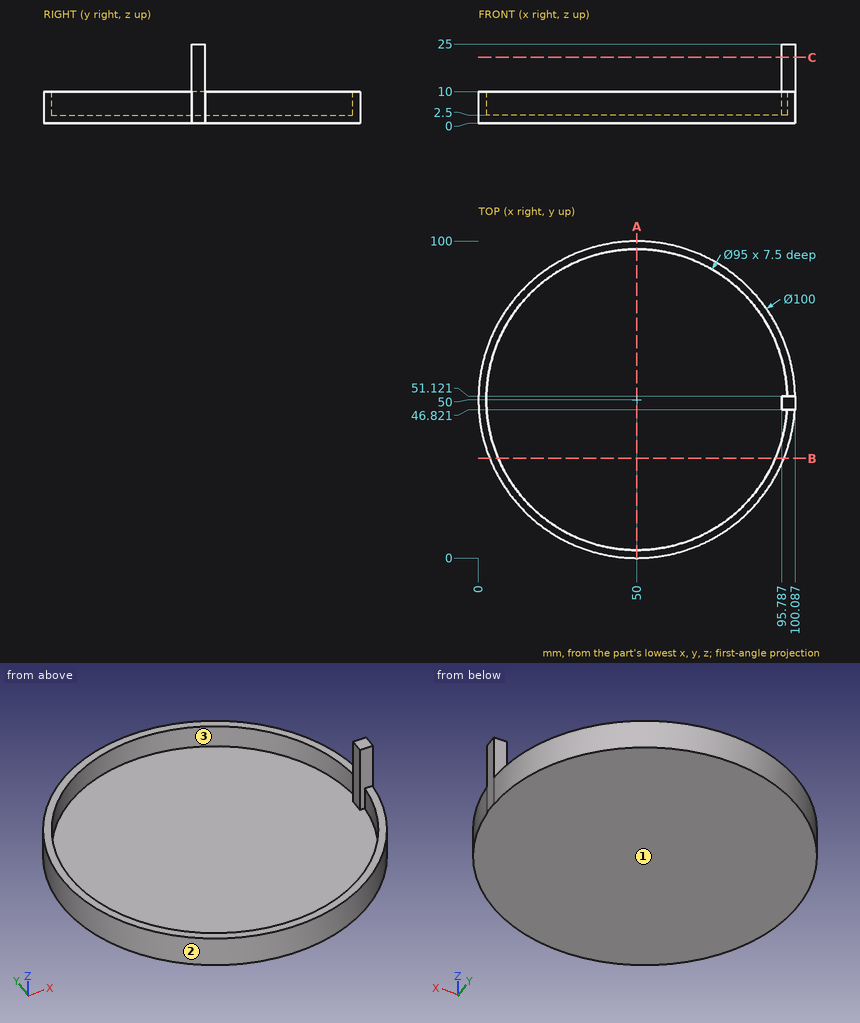
Job drawing, mm, ordinate dimensions from the low corner. One solid piece. Give positions to 0.01 mm unless a question says otherwise; leave off trailing zeros. Order: outer loops, then holes, each group sorted by start corner. A loop starts at its lowest first (then second) coordinate and runs counter-clockwise, first axis right, second up. Notation, with made-up numbers: (52, 41) -> (89, 41) arc R26 ccw to (89, 57) -> close; hole circle Ø7 at (-16, 69.25). An arc over 180 degrees is marked (long way). Return JSON: item names as keys, results as strings.
Q1. Saw through at A-A (x = 50). Write the cut outline in (y, z).
Working result:
{"outline": "(0, 0) -> (100, 0) -> (100, 10) -> (97.5, 10) -> (97.5, 2.5) -> (2.5, 2.5) -> (2.5, 10) -> (0, 10) -> close"}
Q2. Mould opens along Y. For the marked faces 1, 2 and 3 say: pulls with the +Y half, pulls with the -Y half, needs draft (parallel to the pull), parting line crosses it, or undercut.
Working result:
{"face 1": "needs draft", "face 2": "parting line crosses it", "face 3": "undercut"}
Q3. Saw through at B-B (y = 31.5). Write the cut outline in (x, z).
Working result:
{"outline": "(3.55, 0) -> (96.45, 0) -> (96.45, 10) -> (93.75, 10) -> (93.75, 2.5) -> (6.25, 2.5) -> (6.25, 10) -> (3.55, 10) -> close"}
Q4. Drill centre lines: line 1 (X direction, y = 50, z = 4.5); line 2 (Y direction, x = 50, z = 5); line 3 (Z direction, x = 43, y = 24). Where is each one in solid material? Low to high.
Working result:
{"line 1": "0 to 2.5, 95.79 to 100.09", "line 2": "0 to 2.5, 97.5 to 100", "line 3": "0 to 2.5"}
Q5. Saw through at C-C (z = 20.75). Write the cut outline in (x, y), then the cut area to 3 significant figures.
Working result:
{"outline": "(95.79, 46.82) -> (100.09, 46.82) -> (100.09, 51.12) -> (95.79, 51.12) -> close", "area": "18.5 mm²"}
Q6. Flat gauge pins, fed straight in: pin 1 (5 mm diameter, centred on y = 57, z = 3, fed in from -X); pin 2 (1.3 mm diameter, centred on y = 50, z = 17.5, fed in from -X); pin 3 (1 mm diameter, centred on x = 46, y = 23, fed in from +Z). Where does each tip first touch, or does it go through?
Working result:
{"pin 1": "x = 0.2", "pin 2": "x = 95.79", "pin 3": "z = 2.5"}
